The model under review builds one solid part; all positions refer to its coordinate system, in mm. A direction names the side the tool comes from. Round coordinates to 2 decimals unless told otherwise and drop trailing zeros. Write each loop counter-clockwise with the first axis right and the second up, starting at its lowest first coordinate (ties: lowest second). Pieces come first, ordered by that corner, then holes. Notation, with made-up numbers: (54, 76) - (76, 76) arc R31 ccw to (76, 108) - close; hole circle Ø6 at (15, 52). An arc over 180 degrees is marked (long way). Write each question's results on one line, items separated by ' | '.
```python
from build123d import *

# Parameters (mm, degrees)
EXTRUDE_1_DEPTH     = 10
SKETCH_2_W          = 4
SKETCH_2_H          = 17
CUT_EXTRUDE_1_DEPTH = 28.49545417


with BuildPart() as part:
    # 草图1 → 凸台-拉伸1 (new body)
    with BuildSketch(Plane(origin=(0, 0, 0), x_dir=(0, 0, -1), z_dir=(1, 0, 0))):
        with BuildLine():
            Line((2, 0), (18, 0))
            ThreePointArc((18, 0), (19.414213562, -0.585786438), (20, -2))
            Line((20, -2), (20, -14))
            ThreePointArc((20, -14), (19.414213562, -15.414213562), (18, -16))
            Line((18, -16), (9.071485189, -16))
            ThreePointArc((9.071485189, -16), (7.657271627, -15.414213562), (7.071485189, -14))
            Line((7.071485189, -14), (7.071485189, -13))
            Line((7.071485189, -13), (14, -13))
            Line((14, -13), (14, -7))
            Line((14, -7), (4, -7))
            Line((4, -7), (4, -3))
            Line((4, -3), (0, -3))
            Line((0, -3), (0, -2))
            ThreePointArc((0, -2), (0.585786438, -0.585786438), (2, 0))
        make_face()
    extrude(amount=EXTRUDE_1_DEPTH)

    # 草图2 → 切除-拉伸1 (cut, through all)
    with BuildSketch(Plane(origin=(0, 0, 0), x_dir=(1, 0, 0), z_dir=(0, 1, 0))):
        with Locations((5, 11.5)):
            Rectangle(SKETCH_2_W, SKETCH_2_H)
    extrude(amount=-CUT_EXTRUDE_1_DEPTH, mode=Mode.SUBTRACT)


solid = part.part
```
Q1. For probe 1 along X at (y, z) = (-9.5, -16.25); probe 2 along Y at (x, z) = (8.75, -11); probe 3 along Z at (x, y) = (2, -10.75), list the stretches that pass through material, from the lowest coordinate up.
Evaluation:
probe 1: x = 0 to 3, 7 to 10 | probe 2: y = -16 to -13, -7 to 0 | probe 3: z = -20 to -14
Q2. We need section D-D (x = 8.5). State the section outline as (y, z) points.
Evaluation:
outline: (-16, -18) arc R2 ccw to (-14, -20) - (-2, -20) arc R2 ccw to (0, -18) - (0, -2) arc R2 ccw to (-2, 0) - (-3, 0) - (-3, -4) - (-7, -4) - (-7, -14) - (-13, -14) - (-13, -7.07) - (-14, -7.07) arc R2 ccw to (-16, -9.07) - close
Q3. We need section A-A (z = -14.5). State the section outline as (x, y) points.
Evaluation:
outline: (0, -16) - (3, -16) - (3, 0) - (0, 0) - close; (7, -16) - (10, -16) - (10, 0) - (7, 0) - close
Q4. We need section C-C (y = -6). State the section outline as (x, z) points.
Evaluation:
outline: (0, -20) - (3, -20) - (3, -4) - (0, -4) - close; (7, -20) - (10, -20) - (10, -4) - (7, -4) - close
Q5. Tool access review of faces 1 (the flat face through (3, -6, -13)), 2 (the flat face through (8, -5, -4)), 3 (the flat face through (1, -7, -9)): name each direction out of +Z, -Z, +X, -X, +Y, -Y from which nothing blocks a thin tool from reaching the whole face with its end or side.
Evaluation:
face 1: -Z, +Y, -Y | face 2: +Z, +X, -X, -Y | face 3: +Z, +X, -X
Q6. Insertion check: P1, Ø1.1, axis at x = 1, y = -13.5, coming from the +Z side; P2, Ø2.5, axis at x = 8.5, y = -6, coming from the +Z side; P3, Ø2, axis at x = 5, z = -2, coming from the -Y side. Each pin has a flat end and moves straight along its axis. Give the tip position at first contact, or say it passes through.
Evaluation:
P1: stops at z = -7.07 | P2: stops at z = -4 | P3: stops at y = -3
Q7. We need section B-B (z = -12). State the section outline as (x, y) points.
Evaluation:
outline: (0, -16) - (3, -16) - (3, -13) - (0, -13) - close; (0, -7) - (3, -7) - (3, 0) - (0, 0) - close; (7, -16) - (10, -16) - (10, -13) - (7, -13) - close; (7, -7) - (10, -7) - (10, 0) - (7, 0) - close
Q8. The part is to be moulded in two halves that separate along X. For faces 4 (the flat face through (10, -6, -12)), 5 (the flat face through (5, -1, -3)), 6 (the cylindrical face through (4.93, -0.6, -0.57)), say which applies: released by +X, released by -X, zero draft, split by the parting line, or undercut.
Evaluation:
face 4: released by +X | face 5: undercut | face 6: zero draft
